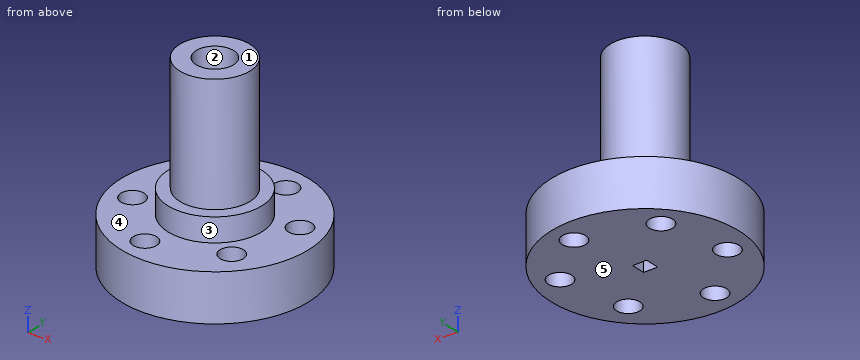
```python
from build123d import *

# Parameters (mm, degrees)
SKETCH1_R           = 20
SKETCH1_R_2         = 2.5
BOSS_EXTRUDE1_DEPTH = 10
SKETCH2_R           = 7.5
BOSS_EXTRUDE2_DEPTH = 30
SKETCH3_R           = 4
CUT_EXTRUDE1_DEPTH  = 30
SKETCH4_W           = 3
SKETCH4_H           = 3
CUT_EXTRUDE2_DEPTH  = 20
SKETCH5_R           = 10
SKETCH5_R_2         = 7.5
BOSS_EXTRUDE3_DEPTH = 5


with BuildPart() as part:
    # Sketch1 → Boss-Extrude1 (new body)
    with BuildSketch(Plane.XY):
        Circle(SKETCH1_R)
        with Locations((3.80920927, 14.508270908)):
            Circle(SKETCH1_R_2, mode=Mode.SUBTRACT)
        with Locations((14.095417524, 5.130224636)):
            Circle(SKETCH1_R_2, mode=Mode.SUBTRACT)
        with Locations((10.763605071, -9.202774002)):
            Circle(SKETCH1_R_2, mode=Mode.SUBTRACT)
        with Locations((-3.511280661, -14.583240659)):
            Circle(SKETCH1_R_2, mode=Mode.SUBTRACT)
        with Locations((-14.415788075, -3.983677546)):
            Circle(SKETCH1_R_2, mode=Mode.SUBTRACT)
        with Locations((-11.178876863, 10.00163547)):
            Circle(SKETCH1_R_2, mode=Mode.SUBTRACT)
    extrude(amount=BOSS_EXTRUDE1_DEPTH)

    # Sketch2 → Boss-Extrude2 (add)
    with BuildSketch(Plane.XY.offset(10)):
        Circle(SKETCH2_R)
    extrude(amount=BOSS_EXTRUDE2_DEPTH)

    # Sketch3 → Cut-Extrude1 (cut)
    with BuildSketch(Plane.XY.offset(40)):
        Circle(SKETCH3_R)
    extrude(amount=-CUT_EXTRUDE1_DEPTH, mode=Mode.SUBTRACT)

    # Sketch4 → Cut-Extrude2 (cut)
    with BuildSketch(Plane(origin=(0, 0, 0), x_dir=(-1, 0, 0), z_dir=(0, 0, -1))):
        Rectangle(SKETCH4_W, SKETCH4_H)
    extrude(amount=-CUT_EXTRUDE2_DEPTH, mode=Mode.SUBTRACT)

    # Sketch5 → Boss-Extrude3 (add)
    with BuildSketch(Plane.XY.offset(10)):
        Circle(SKETCH5_R)
        Circle(SKETCH5_R_2, mode=Mode.SUBTRACT)
    extrude(amount=BOSS_EXTRUDE3_DEPTH)


solid = part.part
```
Here's how the part is built. I have some questions about the finished solid (model axes, mm). Face numbers are marked on the shaded views. A direction names the side the tool comes from. Round coordinates to 2 decimals unless told otherwise and drop trailing zeros. Order: outer loops, then holes, each group sorted by start corner. A loop starts at its lowest first (then second) coordinate and runs counter-clockwise, first axis right, second up. Notation, with made-up numbers: M 0.5,-20 L 53.5,-20 A13 cw 53.5,3 Z; hole C 78,2 d2. An arc over 180 degrees is marked long. Answer in a Markdown table with one row per item.
Item 1: Imagine slicing it at D-D, the plane z = 29. Write out the boundary of the cut face in (x, y).
A:
| item | result |
|---|---|
| outline | C 0,0 d15; hole C 0,0 d8 |
Item 2: Imagine slicing it at C-C, the plane x = -12.5. Write out the boundary of the cut face in (y, z), and give its area (3 significant figures).
A:
| item | result |
|---|---|
| outline | M -15.61,0 L -5.59,0 L -5.59,10 L -15.61,10 Z; M -2.38,0 L 7.88,0 L 7.88,10 L -2.38,10 Z; M 12.12,0 L 15.61,0 L 15.61,10 L 12.12,10 Z |
| area | 238 mm2 |
Item 3: Thinking about a two-plate mould opening in X: for the marked faces 1, 2 and 3, which applies, +X half, -X half, draft (parallel to the pull), parting line (faces both ways), or undercut?
A:
| item | result |
|---|---|
| face 1 | draft |
| face 2 | undercut |
| face 3 | parting line |
Item 4: Imagine slicing it at A-A, the plane x = 0. Write out the boundary of the cut face in (y, z), and give its area (3 significant figures).
A:
| item | result |
|---|---|
| outline | M -20,0 L -1.5,0 L -1.5,10 L -4,10 L -4,40 L -7.5,40 L -7.5,15 L -10,15 L -10,10 L -20,10 Z; M 1.5,0 L 20,0 L 20,10 L 10,10 L 10,15 L 7.5,15 L 7.5,40 L 4,40 L 4,10 L 1.5,10 Z |
| area | 605 mm2 |
Item 5: For the marked faces 4 and 5, which set-ups out of +Z, -Z, +X, -X, +Y, -Y let a thin tool reach every point of the face, with its end or its side?
A:
| item | result |
|---|---|
| face 4 | +Z |
| face 5 | -Z, +X, -X, +Y, -Y |
Item 6: If I drill on L1, parallel to Y at x = 0, z = 28; L2, parallel to Y at x = -2, z = 3; L3, parallel to Z at x = 18.5, y = -2.5, over which ranges is the centre line in solid material (lowest first)? Write a range as from..to.
A:
| item | result |
|---|---|
| L1 | y = -7.5..-4, 4..7.5 |
| L2 | y = -19.9..-16.57, -12.59..19.9 |
| L3 | z = 0..10 |
Item 7: I'm going to push flat-ended pins straight in: pin 1 (4 mm diameter, centred on x = -11.18, y = 10, fed in from +Z); pin 2 (12 mm diameter, centred on y = -0.5, z = 18.5, fed in from -X); pin 3 (12 mm diameter, centred on y = -11, z = 6, fed in from -X); pin 4 (5 mm diameter, centred on x = -10.5, z = 6, fed in from +Y). Where does each tip first touch, or does it pass through?
A:
| item | result |
|---|---|
| pin 1 | passes through |
| pin 2 | stops at x = -10 |
| pin 3 | stops at x = -19.36 |
| pin 4 | stops at y = 18.33 |
